The model under review builds one solid part; all positions refer to its coordinate system, in mm. A direction names the side the tool comes from. Round coordinates to 2 decimals unless told otherwise and drop trailing zeros. Write each loop counter-clockwise with the first axis right and the second up, starting at its lowest first coordinate (ties: lowest second). Pieces come first, ordered by that corner, then holes. Notation, with made-up numbers: (86.5, 89.25) -> (99.5, 89.25) arc R28 ccw to (99.5, 119.25) -> close; hole circle Ø10 at (67, 36). An arc over 180 degrees is marked (long way). Use CSV: the item, a comma, the result in double quotes. Start each with the question number.
1) Take a section at D-D, the plane y = 14.5. Give the boundary of the cut face in (x, z).
2) Take a section at B-B, the plane y = 16.75. Give the boundary of the cut face in (x, z) (3 decimals).
3) Take a section at C-C, the plane y = 4. Give the boundary of the cut face in (x, z) (3 decimals), then the cut area to 3 significant figures.
4) For pin 1 Ø5 at (x, z) = (-4.5, -5) entering from +Y; pin 2 Ø3 at (y, z) = (10.5, 2.5) entering from -X; pin 3 Ø2 at (y, z) = (12, 4.5) entering from +X, all flat-tipped, find the tip position at first contact; note any pin that passes through.
5) Mouldability with a two-part tool opening along X and no side actions: class faces 4 (the face through (0, 11, 0)), 5 (the face through (-2.76, 7.62, 5.93)), 6 (the face through (0, 6, 2.15)), 7 (the face through (0, 21.5, 0)) as released by +X, released by -X, zero draft, split by the parting line, or undercut.
6) Machinability: for faces 1 (the face through (1, 8.25, 7)), 2 (the face through (-1.54, 18.26, 3.72)), 3 (the face through (1.82, 3.65, 5.05)), which of the approach directions +Z, -Z, +X, -X, +Y, -Y give a long, thin tool a straight path to every point of the face, cutting with its end or side? Answer none if there is none.
7) Wall thickness on probe 1 along Z at (x, y) = (0, 8.75) (3 decimals); probe 2 along X at (y, z) = (6.25, 0) (3 decimals); probe 3 along Y at (x, z) = (-4.5, 5.5): over which ranges is each line inside the solid? List them lowest first. Write a range as [from, to].
from build123d import *

# Parameters (mm, degrees)
SKETCH1_R               = 6.05
BOSS_EXTRUDE1_DEPTH     = 7
SKETCH2_R               = 7.2
BOSS_EXTRUDE2_DEPTH     = 1.25
SKETCH3_R               = 7.2
BOSS_EXTRUDE3_DEPTH     = 1.25
SKETCH4_R               = 6.05
BOSS_EXTRUDE4_DEPTH     = 6
CUT_EXTRUDE2_DEPTH      = 19.836570813
CUT_EXTRUDE2_DEPTH_BACK = 11
SKETCH6_R               = 4.025
BOSS_EXTRUDE5_DEPTH     = 6
CHAMFER1_SIZE           = 0.4
CHAMFER2_SIZE           = 0.4


with BuildPart() as part:
    # Sketch1 → Boss-Extrude1 (new body)
    with BuildSketch(Plane(origin=(0, 0, 0), x_dir=(1, 0, 0), z_dir=(0, 1, 0))):
        with Locations(Location((0, 0.72, 0), (0, 0, 270))):
            Circle(SKETCH1_R)
    extrude(amount=BOSS_EXTRUDE1_DEPTH)

    # Sketch2 → Boss-Extrude2 (add)
    with BuildSketch(Plane(origin=(0, 7, 0), x_dir=(1, 0, 0), z_dir=(0, 1, 0))):
        with Locations(Location((0, 0.72, 0), (0, 0, 270))):
            Circle(SKETCH2_R)
    extrude(amount=BOSS_EXTRUDE2_DEPTH)

    # Sketch3 → Boss-Extrude3 (add)
    with BuildSketch(Plane(origin=(0, 8.25, 0), x_dir=(1, 0, 0), z_dir=(0, 1, 0))):
        with Locations(Location((0, -0.72, 0), (0, 0, 174.260829523))):
            Circle(SKETCH3_R)
    extrude(amount=BOSS_EXTRUDE3_DEPTH)

    # Sketch4 → Boss-Extrude4 (add)
    with BuildSketch(Plane(origin=(0, 9.5, 0), x_dir=(1, 0, 0), z_dir=(0, 1, 0))):
        with Locations(Location((0, -0.72, 0), (0, 0, 270))):
            Circle(SKETCH4_R)
    extrude(amount=BOSS_EXTRUDE4_DEPTH)

    # Sketch5 → Cut-Extrude2 (cut, two sides: drawn at the far end of the back side and taken through both)
    with BuildSketch(Plane.XZ.offset(-CUT_EXTRUDE2_DEPTH_BACK)):
        with BuildLine():
            Line((1.506029548, 2.15), (-1.506029548, 2.15))
            ThreePointArc((-1.506029548, 2.15), (0, -2.625), (1.506029548, 2.15))
        make_face()
    extrude(amount=CUT_EXTRUDE2_DEPTH + CUT_EXTRUDE2_DEPTH_BACK, mode=Mode.SUBTRACT)

    # Sketch6 → Boss-Extrude5 (add)
    with BuildSketch(Plane(origin=(0, 15.5, 0), x_dir=(1, 0, 0), z_dir=(0, 1, 0))):
        with Locations(Location((0, 0, 0), (0, 0, 270))):
            Circle(SKETCH6_R)
    extrude(amount=BOSS_EXTRUDE5_DEPTH)

    # Chamfer1
    chamfer1_edges = [part.edges().sort_by_distance(p)[0] for p in [
        (0, 21.5, -4.025),
    ]]
    chamfer(chamfer1_edges, length=CHAMFER1_SIZE)

    # Chamfer2
    chamfer2_edges = [part.edges().sort_by_distance(p)[0] for p in [
        (0, 15.5, -5.33),
        (0, 0, -6.77),
    ]]
    chamfer(chamfer2_edges, length=CHAMFER2_SIZE)


solid = part.part
Values found:
1,outline,"circle Ø12.1 at (0, 0.72)"
2,outline,"circle Ø8.05 at (0, 0)"
3,outline,"circle Ø12.1 at (0, -0.72); hole (-1.506, 2.15) arc R2.625 ccw (long way) to (1.506, 2.15) -> close"
3,area,"94.3 mm²"
4,pin 1,"y = 15.5"
4,pin 2,"x = -7.17"
4,pin 3,"x = 5.37"
5,face 4,"undercut"
5,face 5,"split by the parting line"
5,face 6,"undercut"
5,face 7,"zero draft"
6,face 1,"+Z, -Y"
6,face 2,"+Y"
6,face 3,"-Y"
7,probe 1,"[-6.48, -2.625], [2.15, 7.92]"
7,probe 2,"[-6.007, -2.625], [2.625, 6.007]"
7,probe 3,"[8.25, 9.5]"
